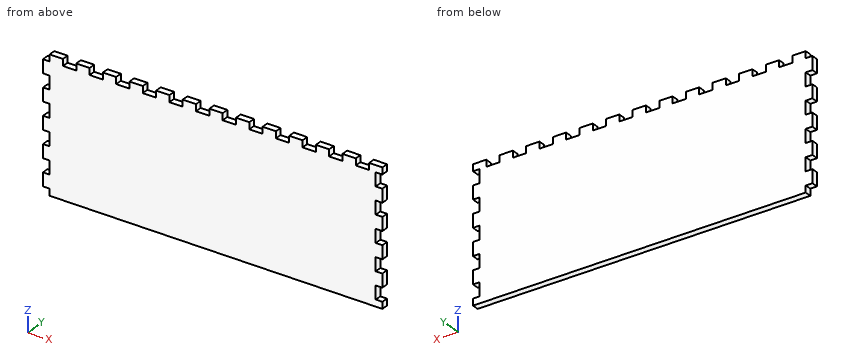
from build123d import *

# Parameters (mm, degrees)
SKETCH013_W             = 95
SKETCH013_H             = 250
PAD011_DEPTH            = 5
SKETCH036_W             = 10
SKETCH036_H             = 5
PAD028_DEPTH            = 5
LINEARPATTERN016_COUNT  = 5
LINEARPATTERN016_PITCH  = 20
SKETCH040_W             = 10
SKETCH040_H             = 5
PAD029_DEPTH            = 5
LINEARPATTERN020_COUNT  = 13
LINEARPATTERN020_PITCH  = 20
SKETCH049_W             = 10
SKETCH049_H             = 5
POCKET015_DEPTH         = 5
LINEARPATTERN029_COUNT  = 5
LINEARPATTERN029_PITCH  = 20
BODY011_PITCH_ANGLE     = -90
BODY011_PLACEMENT_ANGLE = -90


with BuildPart() as part:
    # Sketch013 → Pad011 (new body)
    with BuildSketch(Plane.XY):
        Rectangle(SKETCH013_W, SKETCH013_H)
    extrude(amount=PAD011_DEPTH)

    # Sketch036 (on DatumPlane) → Pad028 (join)
    with BuildSketch(Plane.XZ.offset(125)):
        with Locations((-37.5, 2.5)):
            Rectangle(SKETCH036_W, SKETCH036_H)
    pad028 = extrude(amount=PAD028_DEPTH)

    # LinearPattern016: Pad028 ×5
    with Locations(*[(i * LINEARPATTERN016_PITCH, 0, 0) for i in range(1, LINEARPATTERN016_COUNT)]):
        add(pad028)

    # Sketch040 (on DatumPlane) → Pad029 (join)
    with BuildSketch(Plane.YZ.offset(47.5)):
        with Locations((-120, 2.5)):
            Rectangle(SKETCH040_W, SKETCH040_H)
    pad029 = extrude(amount=PAD029_DEPTH)

    # LinearPattern020: Pad029 ×13
    with Locations(*[(0, i * LINEARPATTERN020_PITCH, 0) for i in range(1, LINEARPATTERN020_COUNT)]):
        add(pad029)

    # Sketch049 (on DatumPlane) → Pocket015 (cut)
    with BuildSketch(Plane(origin=(0, 125, 0), x_dir=(-1, 0, 0), z_dir=(0, 1, 0))):
        with Locations((-42.5, 2.5)):
            Rectangle(SKETCH049_W, SKETCH049_H)
    pocket015 = extrude(amount=-POCKET015_DEPTH, mode=Mode.SUBTRACT)

    # LinearPattern029: Pocket015 ×5
    with Locations(*[(-i * LINEARPATTERN029_PITCH, 0, 0) for i in range(1, LINEARPATTERN029_COUNT)]):
        add(pocket015, mode=Mode.SUBTRACT)


with BuildPart() as part_1:
    # Body011 pitch: moved
    add(part.part.rotate(Axis((0, 0, 0), (0, 1, 0)), BODY011_PITCH_ANGLE))


with BuildPart() as part_2:
    # Body011 placement: moved
    add(part_1.part.moved(Location((-125, -150, 152.5))).rotate(Axis((-125, -150, 152.5), (0, 0, 1)), BODY011_PLACEMENT_ANGLE))


solid = part_2.part
Can you work these out from the model? Positions are in its coordinate system, mm. Give positions to 0.01 mm unless a question says otherwise; leave off trailing zeros. Loops run counter-clockwise (first coordinate to the right, second up) from the corner with the lowest first, then second, coordinate; pieces in that order, holes last. Notation, with made-up numbers: (35, -27.75) -> (91, -27.75) arc R26 ccw to (91, 8.25) -> close; hole circle Ø6 at (20.5, 79.5). An arc over 180 degrees is marked (long way). Return JSON: item names as keys, results as strings.
Q1. I want a section at B-B, the plane x = -213. List the corners of the cut face in (y, z) for me, then the cut area to 3 significant figures.
Checks:
{"outline": "(-150, 105) -> (-145, 105) -> (-145, 200) -> (-150, 200) -> close", "area": "475 mm2"}
Q2. I need wall thicknesses on probe 1 along X at (y, z) = (-147.8, 148); probe 2 along X at (y, z) = (-145.65, 170.5); probe 3 along Z at (x, y) = (-132, -146.7). Which ranges of each line are inside material? Lowest first, please.
Checks:
{"probe 1": "x = -250 to 0", "probe 2": "x = -255 to -5", "probe 3": "z = 105 to 200"}
Q3. For pin 1 Ø1.5 at (x, y) = (-132.5, -148.5) entering from +Z, with a flat end and sliding along its axis, tell me the tip position at first contact or that it passes through.
Checks:
{"pin 1": "stops at z = 200"}
Q4. I want a section at A-A, the plane z = 166. List the corners of the cut face in (x, y) for me, then the cut area to 3 significant figures.
Checks:
{"outline": "(-250, -150) -> (0, -150) -> (0, -145) -> (-250, -145) -> close", "area": "1,250 mm2"}
